Here's the drawing with two shaded views (mm, measured from the low corner). I have some questions. A direction names the side the tool comes from. Coordinates: 2 decimals unless noted, no trailing zeros. Order: outer loops, then holes, each group sorted by start corner. A loop starts at its lowest first (then second) coordinate and runs counter-clockwise, first axis right, second up. Notation, with made-up numbers: M 48.25,-20 L 94.25,-20 A9 ccw 94.25,-7 Z; hole C -31,9 d6. An arc over 180 degrees is marked long. Put each result on its own line as item: value. Start each with the question number.
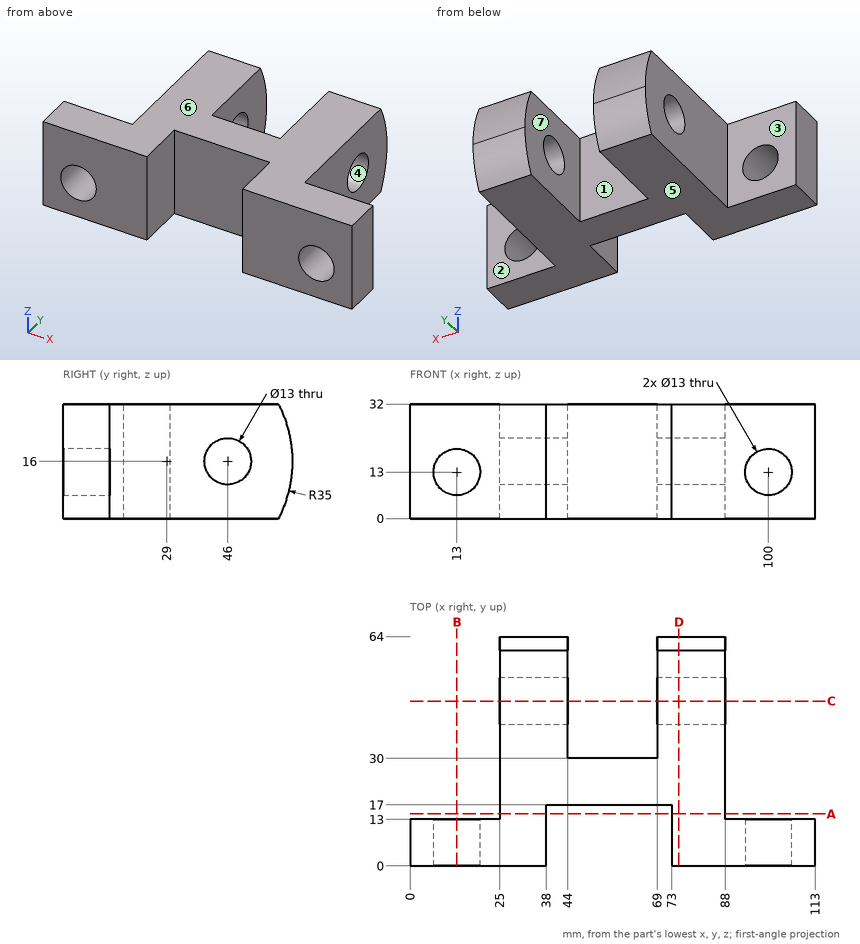
Item 1: I need wall thicknesses on probe 1 along X at (y, z) = (39, 29.5); probe 2 along Z at (x, y) = (39, 46); probe 3 along Z at (x, y) = (32.5, 42). Which ranges of each line are inside material? Lowest first, please.
Item 2: If we section it at B-B on x = 13: Write out the boundary of the cut face in (y, z), then the cut area to 3 significant figures.
Item 3: For pin 1 Ø5 at (x, z) = (45.5, 19) entering from +Y; pin 2 Ø12.5 at (x, z) = (12.5, 11) entering from +Y; pin 3 Ø16 at (x, z) = (51, 8.5) entering from -Y, each with a flat end and sliding along its axis, tell me the tip position at first contact or that it passes through.
Item 4: If we section it at D-D on x = 75: Write out the boundary of the cut face in (y, z).
Item 5: For the marked faces 1, 2 and 3, which set-ups out of +Z, -Z, +X, -X, +Y, -Y let a thin tool reach every point of the face, with its end or its side?
Item 6: If we section it at A-A on y = 14.5: Write out the boundary of the cut face in (x, z).
Item 7: If we section it at C-C on y = 46: Write out the boundary of the cut face in (x, z).
Item 8: If we mould it in two halves opening along Z, with no side actions, what happens to the marked faces 4, 5, 6 and 7? For each: released by +Z, released by -Z, zero draft, split by the parting line, or undercut.
Geometry check:
1. probe 1: x = 25 to 44, 69 to 88
1. probe 2: z = 0 to 9.5, 22.5 to 32
1. probe 3: z = 0 to 10.88, 21.12 to 32
2. outline: M 0,0 L 13,0 L 13,6.5 L 0,6.5 Z; M 0,19.5 L 13,19.5 L 13,32 L 0,32 Z
2. area: 247 mm²
3. pin 1: stops at y = 63.99
3. pin 2: stops at y = 13
3. pin 3: stops at y = 17
4. outline: M 0,0 L 60.13,0 A35 ccw 60.13,32 L 0,32 Z; hole C 46,16 d13
5. face 1: +Z, -Z, +Y
5. face 2: +Z, -Z, +X, +Y
5. face 3: +Z, -Z, -X, +Y
6. outline: M 25,0 L 38,0 L 38,32 L 25,32 Z; M 73,0 L 88,0 L 88,32 L 73,32 Z
7. outline: M 25,0 L 44,0 L 44,9.5 L 25,9.5 Z; M 25,22.5 L 44,22.5 L 44,32 L 25,32 Z; M 69,0 L 88,0 L 88,9.5 L 69,9.5 Z; M 69,22.5 L 88,22.5 L 88,32 L 69,32 Z
8. face 4: undercut
8. face 5: released by -Z
8. face 6: released by +Z
8. face 7: zero draft
